Check sheet for the modelled part. Datum: model origin and axes. Units: mm. A direction names the side the tool comes from. Round coordinates to 2 decimals unless told otherwise and drop trailing zeros. Loops run counter-clockwise (first coordinate to the right, second up) from the corner with the lowest first, then second, coordinate; pieces in that order, holes last. Notation, with made-up numbers: (31.25, 82.25) -> (81.25, 82.25) arc R34 cw to (81.25, 118.25) -> close; hole circle Ø6 at (36.5, 55.5). An arc over 180 degrees is marked (long way). One line per item, written item: value. Start each with the question number.
1. Go/stop test with flat-tipped pins: pin 1 (5.5 mm diameter, centred on x = 0, y = -1, fed in from -Z); pin 2 (1.2 mm diameter, centred on x = -2.5, z = -1, fed in from +Y). Record where each tip stops, or that it passes through.
2. Material ranges on L1, parallel to Z at x = 5, y = 12.5; L2, parallel to Y at x = -3.75, z = -1.1, recorded low to high.
3. Cross-section at B-B on x = -2.5. Record the cut outline in (y, z), then the cut area to 4 significant figures.
4. Set-up check for faces 1 (the face through (9.25, 0, 0)), 2 (the face through (0, 2, -0.5)): record each of +Z, -Z, +X, -X, +Y, -Y from which the full face is reachable in a straight line by a thin tool's end or side.
5. Cross-section at A-A on z = -0.95. Record the cut outline in (x, y), then the cut area to 4 significant figures.
6. Cross-section at C-C on y = 7.5. Record the cut outline in (x, z), then the cut area to 3 significant figures.
from build123d import *

# Parameters (mm, degrees)
F0_W     = 18.5
F0_H     = 39
F1_DEPTH = 0.5
F2_W     = 18.5
F2_H     = 2.5
F3_DEPTH = 1.5


with BuildPart() as f1:
    # F0 (on Top) → F1 (new body, symmetric)
    with BuildSketch(Plane.XY):
        Rectangle(F0_W, F0_H)
    extrude(amount=F1_DEPTH, both=True)

    # F2 (on face) → F3 (join)
    with BuildSketch(Plane(origin=(0, 0, -0.5), x_dir=(1, 0, 0), z_dir=(0, 0, -1))):
        with Locations((0, 18.25)):
            Rectangle(F2_W, F2_H)
    extrude(amount=F3_DEPTH)


solid = f1.part
Taken from the geometry:
1. pin 1: stops at z = -0.5
1. pin 2: stops at y = 19.5
2. L1: z = -0.5 to 0.5
2. L2: y = -19.5 to -17
3. outline: (-19.5, -2) -> (-17, -2) -> (-17, -0.5) -> (19.5, -0.5) -> (19.5, 0.5) -> (-19.5, 0.5) -> close
3. area: 42.75 mm2
4. face 1: +Z, -Z, +X, +Y, -Y
4. face 2: -Z, +X, -X, +Y
5. outline: (-9.25, -19.5) -> (9.25, -19.5) -> (9.25, -17) -> (-9.25, -17) -> close
5. area: 46.25 mm2
6. outline: (-9.25, -0.5) -> (9.25, -0.5) -> (9.25, 0.5) -> (-9.25, 0.5) -> close
6. area: 18.5 mm2
